```python
from build123d import *

# Parameters (mm, degrees)
F0_W      = 41
F0_H      = 41
F1_DEPTH  = 43
F2_W      = 41
F2_H      = 9
F3_DEPTH  = 12.7
F5_DEPTH  = 4
F6_R      = 6.35
F7_R      = 1.60019
F8_R      = 1.6002
F9_R      = 0.7874
F11_DEPTH = 8
F12_W     = 41
F12_H     = 41
F13_DEPTH = 21
F15_D     = 2.3876
F15_DEPTH = 12.7
F15_TIP   = 0.717307407
F16_R     = 1.9812
F17_DEPTH = 2.3876
F18_R     = 3.175
F19_DEPTH = 3.9624
F21_DEPTH = 4.7752
F23_R     = 3.175
F24_DEPTH = 21.7254
F28_W     = 21
F28_H     = 25.4
F29_DEPTH = 15.875
F30_R     = 5.08
F32_DEPTH = 6


# Not quite as in the source:
# - a fillet or chamfer is up to 0.001 mm smaller than in the source, because OpenCascade refuses the exact size


with BuildPart() as f1:
    # F0 (on Front) → F1 (new body)
    with BuildSketch(Plane.XZ):
        Rectangle(F0_W, F0_H)
    extrude(amount=F1_DEPTH)

    # F2 (on face) → F3 (join)
    with BuildSketch(Plane.XZ.offset(43)):
        with Locations((0, -16)):
            Rectangle(F2_W, F2_H)
    extrude(amount=F3_DEPTH)

    # F4 (on face) → F5 (join)
    with BuildSketch(Plane.XZ.offset(43)):
        with BuildLine():
            Line((-22.0036495704, 24.0950572902), (-20.4869841684, 0.4436360632))
            ThreePointArc((-20.4869841684, 0.4436360632), (-13.7436360632, -5.4869841684), (-7.8130158316, 1.2563639368))
            Line((-7.8130158316, 1.2563639368), (-8.6257437052, 13.9303322737))
            Line((-8.6257437052, 13.9303322737), (29.5957513579, 16.3813147587))
            Line((29.5957513579, 16.3813147587), (29.4429585176, 18.764020806))
            Line((29.4429585176, 18.764020806), (21.5090543388, 18.2552531571))
            Line((21.5090543388, 18.2552531571), (20.9579096507, 26.85))
            Line((20.9579096507, 26.85), (-22.0036495704, 24.0950572902))
        make_face()
    extrude(amount=F5_DEPTH)

    # F6
    f6_edges = [f1.edges().sort_by_distance(p)[0] for p in [
        (21.509054, -45, 18.255253),
    ]]
    fillet(f6_edges, radius=F6_R)

    # F7 (radius 1.6002 in the source; OpenCascade refuses exactly that, so slightly less here)
    f7_edges = [f1.edges().sort_by_distance(p)[0] for p in [
        (29.442959, -45, 18.764021),
    ]]
    fillet(f7_edges, radius=F7_R)

    # F8
    f8_edges = [f1.edges().sort_by_distance(p)[0] for p in [
        (20.95791, -45, 26.85),
    ]]
    fillet(f8_edges, radius=F8_R)

    # F9
    f9_edges = [f1.edges().sort_by_distance(p)[0] for p in [
        (29.595751, -45, 16.381315),
    ]]
    fillet(f9_edges, radius=F9_R)

    # F10 (on face) → F11 (join)
    with BuildSketch(Plane.XZ.offset(47)):
        with BuildLine():
            Line((19.3609896402, 26.7475962879), (-22.0036495704, 24.0950572902))
            Line((-22.0036495704, 24.0950572902), (-21.2997120421, 13.1176044))
            Line((-21.2997120421, 13.1176044), (-8.6257437052, 13.9303322737))
            Line((-8.6257437052, 13.9303322737), (28.809965321, 16.3309256305))
            ThreePointArc((28.809965321, 16.3309256305), (29.3508413223, 16.5967075264), (29.5453622297, 17.1671007956))
            ThreePointArc((29.5453622297, 17.1671007956), (29.0052248284, 18.2663004111), (27.8460385072, 18.661617094))
            ThreePointArc((27.8460385072, 18.661617094), (23.246092788, 20.2303340893), (21.102690402, 24.5922373256))
            Line((21.102690402, 24.5922373256), (21.0603133628, 25.2530799896))
            ThreePointArc((21.0603133628, 25.2530799896), (20.5201759615, 26.3522796051), (19.3609896402, 26.7475962879))
        make_face()
    extrude(amount=F11_DEPTH)

    # F12 (on face) → F13 (join)
    with BuildSketch(Plane.XZ.offset(55.7)):
        Rectangle(F12_W, F12_H)
    extrude(amount=F13_DEPTH)

    # F15
    with Locations(Plane(origin=(-1.628897193, 0, 25.4016038063), x_dir=(0.9979502627, 0, 0.0639943208), z_dir=(-0.0639943208, 0, 0.9979502627))):
        with Locations((-6.1164010452, -50)):
            Hole(F15_D / 2, depth=F15_DEPTH)
            with Locations((0, 0, -(F15_DEPTH + F15_TIP / 2))):  # 118° drill point
                Cone(0, F15_D / 2, F15_TIP, mode=Mode.SUBTRACT)

    # F16 (on face) → F17 (join)
    with BuildSketch(Plane(origin=(-1.628897193, 0, 25.4016038063), x_dir=(0.9979502627, 0, 0.0639943208), z_dir=(-0.0639943208, 0, 0.9979502627))):
        with Locations((12.1207989548, -49)):
            Circle(F16_R)
    extrude(amount=F17_DEPTH)

    # F18 (on face) → F19 (join)
    with BuildSketch(Plane(origin=(-1.7816900333, 0, 27.7843098536), x_dir=(0.9979502627, 0, 0.0639943208), z_dir=(-0.0639943208, 0, 0.9979502627))):
        with Locations((12.1207989548, -49)):
            Circle(F18_R)
    extrude(amount=F19_DEPTH)

    # F20 (on face) → F21 (join)
    with BuildSketch(Plane(origin=(0, 0, -20.5), x_dir=(1, 0, 0), z_dir=(0, 0, -1))):
        Polygon((-5.7375, 43), (-0.975, 45.749630657), (-0.975, 51.248891971), (-5.7375, 53.9985226281), (-10.5, 51.248891971), (-10.5, 45.749630657), align=None)
    extrude(amount=F21_DEPTH)

    # F23 (on offset) → F24 (join, through all)
    with BuildSketch(Plane(origin=(0, 0, -26.8754), x_dir=(1, 0, 0), z_dir=(0, 0, -1))):
        with Locations((-5.7375, 48.499261314)):
            Circle(F23_R)
    extrude(amount=-F24_DEPTH)

    # F26 (on face) → F27 (revolve)
    with BuildSketch(Plane(origin=(-14.15, 0, 0), x_dir=(0, -1, 0), z_dir=(-1, 0, 0))):
        with BuildLine():
            Line((47.7874, 5.6128158316), (47, 5.6128158316))
            Line((47, 5.6128158316), (47, 0.8630158316))
            Line((47, 0.8630158316), (51.3688, 0.8630158316))
            Line((51.3688, 0.8630158316), (51.3688, 7.2130158316))
            Line((51.3688, 7.2130158316), (50.5814, 7.2130158316))
            ThreePointArc((50.5814, 7.2130158316), (49.5781, 6.392545411), (48.5748, 7.2130158316))
            Line((48.5748, 7.2130158316), (47.7874, 7.2130158316))
            Line((47.7874, 7.2130158316), (47.7874, 5.6128158316))
        make_face()
    revolve(axis=Axis((-14.15, -49.1844, 0.8630158316), (0, -1, 0)))

    # F28 (on face) → F29 (join)
    with BuildSketch(Plane(origin=(0, 0, -26.8754), x_dir=(1, 0, 0), z_dir=(0, 0, -1))):
        with Locations((-5.5, 44)):
            Rectangle(F28_W, F28_H)
    extrude(amount=F29_DEPTH)

    # F30
    f30_edges = [f1.edges().sort_by_distance(p)[0] for p in [
        (-5.5, -56.7, -42.7504),
        (-5.5, -56.7, -26.8754),
        (-5.5, -31.3, -42.7504),
        (-5.5, -31.3, -26.8754),
    ]]
    fillet(f30_edges, radius=F30_R)

    # F31 (on face) → F32 (join)
    with BuildSketch(Plane(origin=(0, 0, -42.7504), x_dir=(1, 0, 0), z_dir=(0, 0, -1))):
        Polygon((-4.0054491924, 45.499261314), (-2.2733983849, 48.499261314), (-4.0054491924, 51.499261314), (-7.4695508076, 51.499261314), (-9.2016016151, 48.499261314), (-7.4695508076, 45.499261314), align=None)
    extrude(amount=F32_DEPTH)

    # F34 (on offset) → F35 (revolve, cut)
    with BuildSketch(Plane.XZ.offset(48.502061314)):
        Polygon((-2.2479983849, -44.7504), (-5.4875, -48.7504), (-2.2479983849, -48.7504), align=None)
    revolve(axis=Axis((-5.7375, -48.502061314, -47.4463791664), (0, 0, 1)), mode=Mode.SUBTRACT)


solid = f1.part
```
Work out the finished part from the listing and answer in its coordinate system (mm). A direction names the side the tool comes from. Round coordinates to 2 decimals unless told otherwise and drop trailing zeros. Order: outer loops, then holes, each group sorted by start corner. A loop starts at its lowest first (then second) coordinate and runs counter-clockwise, first axis right, second up.
Q1. A cutting plane is placed at A-A, the plane y = -39.5. Determine the outline of the cut face in (x, z).
Solution:
outline: (-20.5, -20.5) - (20.5, -20.5) - (20.5, 20.5) - (-20.5, 20.5) - close; (-16, -42.75) - (5, -42.75) - (5, -26.88) - (-16, -26.88) - close
Q2. The mould has two halves that part along Y. Classify faces 1 (the flat face through (-3.15, -46.98, -44.03)), 2 (the cylindrical face through (-20.446, -48.176, 0.036)), 3 (the flat face through (5, -44, -35)), 4 (the flat face through (-14, -51.369, 1)): pulls with the +Y half, pulls with the -Y half, needs draft (parallel to the pull), parting line crosses it, or undercut.
Solution:
face 1: pulls with the +Y half
face 2: undercut
face 3: needs draft
face 4: undercut
Q3. Given pin 1 Ø4.5 at (x, y) = (-6, -44) entering from +Z; pin 2 Ø7.5 at (x, y) = (-10.5, -46.5) entering from -Z; pin 3 Ø5 at (y, z) = (-42, -37.5) entering from -X, each flat-ended and moving along its own axis, determine where each tip first touches the part or whether it passes through.
Solution:
pin 1: stops at z = 25.27
pin 2: stops at z = -47.31
pin 3: stops at x = -16
Q4. Find the intervals of material crossed by line 1 along Y through (x, z) = (-16, 6); line 2 along Y through (x, z) = (-6, 11.5); line 3 along Y through (x, z) = (-2, 15), in increasing order.
Solution:
line 1: y = -76.7 to -55.7, -51.37 to -47.79, -47 to 0
line 2: y = -76.7 to -55.7, -43 to 0
line 3: y = -76.7 to -55.7, -55 to 0
Q5. A cutting plane is placed at D-D, the plane y = -62. Determine the outline of the cut face in (x, z), then the cut area to 3 significant figures.
Solution:
outline: (-20.5, -20.5) - (20.5, -20.5) - (20.5, 20.5) - (-20.5, 20.5) - close
area: 1,680 mm2
Q6. A tool of negligible diameter and unlimited length cuts with its end or side. For faces 5 (the flat face through (0, -21, 20.5)), 6 (the flat face through (-3.323, -52.604, -22.854)), 7 (the flat face through (-6, -51.499, -44)), from which of +Z, -Z, +X, -X, +Y, -Y can it reach the whole face along a straight path? Write none if from no direction.
Solution:
face 5: +Z, +X, -X, +Y
face 6: +X, -Y
face 7: -Z, +X, -X, -Y
Q7. A cutting plane is placed at B-B, the plane z = -8. Count the separate pieces of the cut face and the enclosed holes in it, then the cut area to 3 significant figures.
Solution:
separate pieces: 3
enclosed holes: 0
area: 2,660 mm2
